Read the model definition and answer for the solid it produces. Units are mm, in the model's axes. A direction names the side the tool comes from. Coordinates: 2 decimals unless noted, no trailing zeros. Write each loop counter-clockwise with the first axis right and the second up, starting at its lowest first coordinate (ties: lowest second). Pieces come first, ordered by that corner, then holes. Notation, with made-up numbers: M -6.5,24 L 39.5,24 A24 cw 39.5,60 Z; hole C -7,-34.75 d6. An arc over 180 degrees is marked long. Use a Markdown table: item, result. Add a question column.
from build123d import *

# Parameters (mm, degrees)
F0_W        = 35
F0_H        = 35
F1_DEPTH    = 15
F3_R        = 4.5
F4_DEPTH    = 3
F5_T1_DEPTH = 3.9749724421
F6_R        = 5


# Not quite as in the source:
# - a fillet or chamfer that OpenCascade refuses, or shapes differently, is made with other operations: its cross-section is extruded or revolved along the edge and cut away or added


with BuildPart() as f1:
    # F0 (on Front) → F1 (new body, symmetric)
    with BuildSketch(Plane.XZ):
        Rectangle(F0_W, F0_H)
    extrude(amount=F1_DEPTH, both=True)

    # F3 (on face) → F4 (join)
    with BuildSketch(Plane.XZ.offset(15)):
        with BuildLine():
            Line((-12.0646512398, 3), (-12.0646512398, 0))
            Line((-12.0646512398, 0), (-12.0646512398, -3))
            ThreePointArc((-12.0646512398, -3), (-7.6541876394, -6.4685364284), (-6.7129943114, -12))
            Line((-6.7129943114, -12), (-0.7129943114, -12))
            ThreePointArc((-0.7129943114, -12), (-2.1988842528, -5.1949035825), (-6.8389470689, 0))
            ThreePointArc((-6.8389470689, 0), (-2.1988842528, 5.1949035825), (-0.7129943114, 12))
            Line((-0.7129943114, 12), (-6.7129943114, 12))
            ThreePointArc((-6.7129943114, 12), (-7.6541876394, 6.4685364284), (-12.0646512398, 3))
        make_face()
        with BuildLine():
            Line((11.0439136906, 12), (11.0439136906, 6.6378525317))
            ThreePointArc((11.0439136906, 6.6378525317), (-0.6094940203, -3.5115698933), (14.5591460332, -0.5577510491))
            Line((14.5591460332, -0.5577510491), (14.5439136906, -0.5577510491))
            Line((14.5439136906, -0.5577510491), (14.5439136906, 12))
            Line((14.5439136906, 12), (11.0439136906, 12))
        make_face()
        with Locations((6.578612607, 0)):
            Circle(F3_R, mode=Mode.SUBTRACT)
    extrude(amount=F4_DEPTH)

    # F5: fillet of radius 5 on 1 edges, made by hand

    # F5_s2 → F5_t1 (join)
    with BuildSketch(Plane.XZ.offset(14.0250275579)):
        with BuildLine():
            ThreePointArc((14.5591460332, -0.5577510491), (14.5477232275, -0.3629052417), (14.5439136906, -0.1677620723))
            Line((14.5439136906, -0.1677620723), (14.5439136906, -0.5577510491))
            Line((14.5439136906, -0.5577510491), (14.5591460332, -0.5577510491))
        make_face()
    extrude(amount=F5_T1_DEPTH)

    # F6
    f6_edges = [f1.edges().sort_by_distance(p)[0] for p in [
        (14.559146, -16.5, -0.557751),
    ]]
    fillet(f6_edges, radius=F6_R)


solid = f1.part
Item 1: Each of these flat-tipped pins is pushed along its axis until it touches: pin 1 (0.9 mm diameter, centred on y = -16, z = 1.5, fed in from -X); pin 2 (1 mm diameter, centred on x = -12, z = 10, fed in from -Y); pin 3 (0.9 mm diameter, centred on y = -16.5, z = 10, fed in from -X). Where does it stop, or does it pass through?
Item 2: Determine the mould class of faces 6 (the cylindrical face through (-7.696, -16.479, -6.4)), 7 (the cylindrical face through (-2.154, -16.479, -5.283)), 8 (the flat face through (0, 0, 17.5)) for opening direction X: pulls with the +X half, pulls with the -X half, needs draft (parallel to the pull), parting line crosses it, or undercut.
Item 3: Find section A-A on x = 12. Give the vertices of the cut face in (y, z).
Item 4: Find section B-B on z = -11.5. Give the vertices of the cut face in (x, y), then the cut area to 3 significant figures.
Item 5: Consider probe 1 along Y at (x, z) = (-9.5, 7.5); probe 2 along Z at (x, y) = (12.5, -15.5). Determine where each line is inside the solid, lowest interval first.
Item 6: Find section D-D on z = 4. Give the vertices of the cut face in (x, y).
Item 7: For faces 1 (the flat face through (-12.065, -16, 0)), 2 (the cylindrical face through (-7.61, -16.48, 6.54)), 3 (the flat face through (13, -16, 12)), 4 (the flat face through (11.044, -16, 9)), 5 (the cylindrical face through (5.99, -16.48, 4.46)), determine the directions among +Z, -Z, +X, -X, +Y, -Y from which every point of the face is accessible in a straight line to the end or side of a thin tool.
Item 8: Find section C-C on x = 4. Give the vertices of the cut face in (y, z).
Geometry says:
| question | item | result |
|---|---|---|
| 1 | pin 1 | stops at x = -12.06 |
| 1 | pin 2 | stops at y = -15 |
| 1 | pin 3 | stops at x = -6.61 |
| 2 | face 6 | pulls with the -X half |
| 2 | face 7 | undercut |
| 2 | face 8 | needs draft |
| 3 | outline | M -18,-5.88 L -15,-5.88 L -15,-17.5 L 15,-17.5 L 15,17.5 L -15,17.5 L -15,12 L -18,12 Z |
| 4 | outline | M -17.5,-15 L -6.63,-15 L -6.63,-18 L -0.7,-18 L -0.7,-15 L 17.5,-15 L 17.5,15 L -17.5,15 Z |
| 4 | area | 1,070 mm2 |
| 5 | probe 1 | y = -15 to 15 |
| 5 | probe 2 | z = -5.38 to 12 |
| 6 | outline | M -17.5,-15 L -9.98,-15 L -9.98,-18 L -2.89,-18 L -2.89,-15 L -0.35,-15 L -0.35,-18 L 4.52,-18 L 4.52,-15 L 8.64,-15 L 8.64,-18 L 14.54,-18 L 14.54,-15 L 17.5,-15 L 17.5,15 L -17.5,15 Z |
| 7 | face 1 | +Z, -Z, -X, -Y |
| 7 | face 2 | -X, -Y |
| 7 | face 3 | +Z, +X, -X, -Y |
| 7 | face 4 | +Z, -Y |
| 7 | face 5 | -Y |
| 8 | outline | M -18,-7.57 L -15,-7.57 L -15,-17.5 L 15,-17.5 L 15,17.5 L -15,17.5 L -15,7.57 L -18,7.57 L -18,3.69 L -15,3.69 L -15,-3.69 L -18,-3.69 Z |
